CAD build for the part. Positions are in the model's coordinates, mm. Face numbers are marked on the shaded views. A direction names the side the tool comes from. Round coordinates to 2 decimals unless told otherwise and drop trailing zeros. Write each loop counter-clockwise with the first axis right and the second up, starting at its lowest first coordinate (ties: lowest second). Pieces come first, ordered by that corner, then holes. Notation, with made-up numbers: (12.25, 56) -> (71.25, 56) arc R29 cw to (71.25, 94) -> close; hole circle Ø2 at (70, 88). An arc over 180 degrees is marked (long way). Answer in a Markdown table with one row per item. Add a question column.
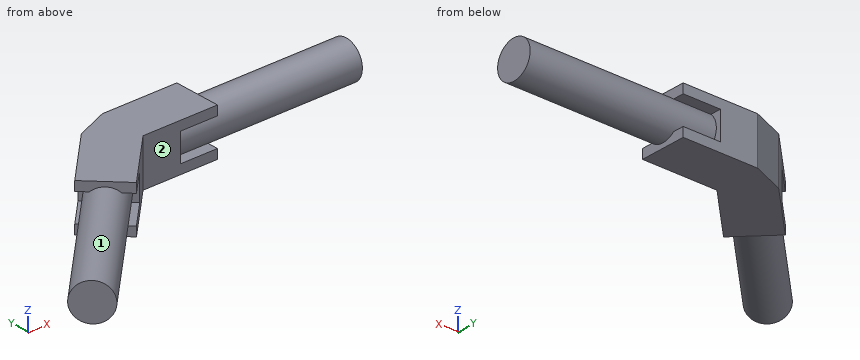
```python
from build123d import *

# Parameters (mm, degrees)
SKETCH1_R           = 12.7
BOSS_EXTRUDE1_DEPTH = 127
SKETCH2_W           = 31.75
SKETCH2_H           = 31.75
BOSS_EXTRUDE2_DEPTH = 25.4
SKETCH3_W           = 25.4
SKETCH3_H           = 31.75
BOSS_EXTRUDE3_DEPTH = 6.35
SKETCH4_W           = 25.4
SKETCH4_H           = 31.75
BOSS_EXTRUDE4_DEPTH = 6.35
SKETCH9_W           = 31.75
SKETCH9_H           = 31.75
BOSS_EXTRUDE5_DEPTH = 25.4
SKETCH11_R          = 12.7
BOSS_EXTRUDE6_DEPTH = 127
BOSS_EXTRUDE7_DEPTH = 6.35
BOSS_EXTRUDE8_DEPTH = 6.35
BOSS_EXTRUDE9_DEPTH = 31.75


with BuildPart() as part:
    # Sketch1 → Boss-Extrude1 (new body)
    with BuildSketch(Plane(origin=(0, 0, 0), x_dir=(0, 0, -1), z_dir=(1, 0, 0))):
        Circle(SKETCH1_R)
    extrude(amount=BOSS_EXTRUDE1_DEPTH)

    # Sketch2 → Boss-Extrude2 (add)
    with BuildSketch(Plane.ZY):
        Rectangle(SKETCH2_W, SKETCH2_H)
    extrude(amount=BOSS_EXTRUDE2_DEPTH)

    # Sketch3 → Boss-Extrude3 (add)
    with BuildSketch(Plane.XY.offset(15.875)):
        with Locations((12.7, 0)):
            Rectangle(SKETCH3_W, SKETCH3_H)
    extrude(amount=-BOSS_EXTRUDE3_DEPTH)

    # Sketch4 → Boss-Extrude4 (add)
    with BuildSketch(Plane(origin=(0, 0, -15.875), x_dir=(-1, 0, 0), z_dir=(0, 0, -1))):
        with Locations((-12.7, 0)):
            Rectangle(SKETCH4_W, SKETCH4_H)
    extrude(amount=-BOSS_EXTRUDE4_DEPTH)



with BuildPart() as body_2:
    # Sketch9 → Boss-Extrude5 (new body)
    with BuildSketch(Plane(origin=(-20.6375, -20.6375, 0), x_dir=(0, 0, 1), z_dir=(-0.707106781, -0.707106781, 0))):
        with Locations((0, 22.610192091)):
            Rectangle(SKETCH9_W, SKETCH9_H)
    extrude(amount=BOSS_EXTRUDE5_DEPTH)

    # Sketch11 → Boss-Extrude6 (add)
    with BuildSketch(Plane(origin=(-38.598012242, -38.598012242, 0), x_dir=(0, 0, 1), z_dir=(-0.707106781, -0.707106781, 0))):
        with Locations((0, 22.610192091)):
            Circle(SKETCH11_R)
    extrude(amount=BOSS_EXTRUDE6_DEPTH)

    # Sketch13 → Boss-Extrude7 (add)
    with BuildSketch(Plane.XY.offset(15.875)):
        Polygon((-43.360512242, -33.835512242), (-61.321024484, -51.796024484), (-83.771664787, -29.345384182), (-65.811152545, -11.384871939), align=None)
    extrude(amount=-BOSS_EXTRUDE7_DEPTH)

    # Sketch14 → Boss-Extrude8 (add)
    with BuildSketch(Plane(origin=(0, 0, -15.875), x_dir=(-1, 0, 0), z_dir=(0, 0, -1))):
        Polygon((65.811152545, -11.384871939), (83.771664787, -29.345384182), (61.321024484, -51.796024484), (43.360512242, -33.835512242), align=None)
    extrude(amount=-BOSS_EXTRUDE8_DEPTH)


with BuildPart() as part_1:
    add(part.part)

    add(body_2.part)  # Boss-Extrude9 merges body 2
    # Sketch15 → Boss-Extrude9 (add)
    with BuildSketch(Plane(origin=(0, 0, -15.875), x_dir=(-1, 0, 0), z_dir=(0, 0, -1))):
        Polygon((25.4, 15.875), (47.850640303, 6.575640303), (25.4, -15.875), align=None)
    extrude(amount=-BOSS_EXTRUDE9_DEPTH)


solid = part_1.part
```
Item 1: Saw through at D-D on x = 97. Give the cut face in (y, z).
Item 2: Tool access for the marked faces 1 and 2: list every direction of +Z, -Z, +X, -X, +Y, -Y with a clear straight run to the whole face (end or side of a thin tool).
Item 3: Drill centre lines: probe 1 along Y at (x, z) = (-23.5, 12) (3 decimals); probe 2 along Y at (x, z) = (-61.5, 7); probe 3 along Z at (x, y) = (-104, -68). Where is each one in solid material? Low to high.
Item 4: Saw through at C-C on z = 7. Give the cut face in (x, y) (3 decimals), then the cut area to 3 significant figures.
Item 5: Pin check, flat tips, straight feed: pin 1 (9.5 mm diameter, centred on x = 9.5, z = -1.5, fed in from -Y); pin 2 (8 mm diameter, centred on x = -72.5, z = 11, fed in from +Y); pin 3 (2 mm diameter, centred on y = 13, z = -3, fed in from +X); pin 4 (6 mm diameter, centred on x = -82, z = 11, fed in from -Y). Stop position of each tip, or through.
Item 6: Saw through at B-B on y = -5. Give the cut face in (x, z) (3 decimals), then the cut area to 3 significant figures.
Item 7: Saw through at A-A on x = 8.5. Give the cut face in (y, z) (3 decimals), then the cut area to 3 significant figures.
Recorded:
| question | item | result |
|---|---|---|
| 1 | outline | circle Ø25.4 at (0, 0) |
| 2 | face 1 | none |
| 2 | face 2 | +Z, -Z, +X, -Y |
| 3 | probe 1 | -15.875 to 15.875 |
| 3 | probe 2 | -44.51 to -7.07 |
| 3 | probe 3 | -12.38 to 12.38 |
| 4 | outline | (-151.881, -104.92) -> (-136.895, -119.906) -> (-47.093, -30.103) -> (-43.361, -33.836) -> (-25.4, -15.875) -> (0, -15.875) -> (0, -10.597) -> (127, -10.597) -> (127, 10.597) -> (0, 10.597) -> (0, 15.875) -> (-25.4, 15.875) -> (-47.851, 6.576) -> (-65.811, -11.385) -> (-62.079, -15.117) -> close |
| 4 | area | 7,350 mm2 |
| 5 | pin 1 | y = -12.7 |
| 5 | pin 2 | y = -14.07 |
| 5 | pin 3 | x = 127 |
| 5 | pin 4 | y = -65.04 |
| 6 | outline | (-59.426, -15.875) -> (25.4, -15.875) -> (25.4, -11.674) -> (127, -11.674) -> (127, 11.674) -> (25.4, 11.674) -> (25.4, 15.875) -> (-59.426, 15.875) -> close |
| 6 | area | 5,070 mm2 |
| 7 | outline | (-15.875, -15.875) -> (15.875, -15.875) -> (15.875, -9.525) -> (8.4, -9.525) arc R12.7 ccw to (8.4, 9.525) -> (15.875, 9.525) -> (15.875, 15.875) -> (-15.875, 15.875) -> (-15.875, 9.525) -> (-8.4, 9.525) arc R12.7 ccw to (-8.4, -9.525) -> (-15.875, -9.525) -> close |
| 7 | area | 837 mm2 |
